from build123d import *

# Parameters (mm, degrees)
F0_R     = 26.071284
F1_DEPTH = 25.4


with BuildPart() as f1:
    # F0 (on Front) → F1 (new body)
    with BuildSketch(Plane.XZ):
        with BuildLine():
            Line((-40.295284, 43.9585), (-40.295284, -43.9585))
            Line((-40.295284, -43.9585), (40.295284, -43.9585))
            Line((40.295284, -43.9585), (40.295284, 43.9585))
            ThreePointArc((40.295284, 43.9585), (0, 3.663216), (-40.295284, 43.9585))
        make_face()
        with BuildLine():
            ThreePointArc((40.295284, 43.9585), (0, 84.253784), (-40.295284, 43.9585))
            ThreePointArc((-40.295284, 43.9585), (0, 3.663216), (40.295284, 43.9585))
        make_face()
        with Locations((0, 43.9585)):
            Circle(F0_R, mode=Mode.SUBTRACT)
    extrude(amount=F1_DEPTH)


solid = f1.part
Geometry: final body of the model. Coordinates: model frame, mm. Round coordinates to 2 decimals unless told otherwise and drop trailing zeros. Loops run counter-clockwise (first coordinate to the right, second up) from the corner with the lowest first, then second, coordinate; pieces in that order, holes last. Notation, with made-up numbers: M 7.25,-13.5 L 52.25,-13.5 A15 ccw 52.25,13.5 Z; hole C 47,-24 d2. An arc over 180 degrees is marked long. One line per question, with ' | ' between items.
(1) Cut plane D-D on x = 29. Return the cut outline in (y, z).
Check result:
outline: M -25.4,-43.96 L 0,-43.96 L 0,71.94 L -25.4,71.94 Z
(2) Cut plane C-C on y = -20.75. Return the cut outline in (x, z), plus the area to 3 significant figures.
Check result:
outline: M -40.3,-43.96 L 40.3,-43.96 L 40.3,43.96 A40.3 ccw -40.3,43.96 Z; hole C 0,43.96 d52.14 | area: 7,500 mm2
(3) Material intervals for line 1 along X through (y, z) = (-1.5, 43); line 2 along Z through (x, y) = (0, -11); line 3 along Z through (x, y) = (12, -14), sorted ascending. Write a range as from..to.
Check result:
line 1: x = -40.3..-26.05, 26.05..40.3 | line 2: z = -43.96..17.89, 70.03..84.25 | line 3: z = -43.96..20.81, 67.1..82.43
(4) Cut plane B-B on z = 21. Return the cut outline in (x, y), plus the area to 3 significant figures.
Check result:
outline: M -40.3,-25.4 L -12.35,-25.4 L -12.35,0 L -40.3,0 Z; M 12.35,-25.4 L 40.3,-25.4 L 40.3,0 L 12.35,0 Z | area: 1,420 mm2
(5) Pull-direction query (Z, two-part tool) for faces 1 (the flat face through (-1, -13, -43.958)), 2 (the flat face through (-1, 0, 7)), 3 (the cylindrical face through (14.02, -12.52, 65.94)); classes: +Z half, -Z half, draft (parallel to the pull), parting line (faces both ways), or undercut.
Check result:
face 1: -Z half | face 2: draft | face 3: undercut
(6) Contact query for flat-ended pins moving along their axis: P1, Ø2, axis at x = 26.5, y = -12, coming from the +Z side; P2, Ø1.5, axis at x = -31.5, y = -11.5, coming from the +Z side; P3, Ø12, axis at x = -31, y = -13.5, coming from the +Z side. Output: stop coordinate, or through.
Check result:
P1: stops at z = 75.16 | P2: stops at z = 70 | P3: stops at z = 75.56
(7) Cut plane A-A on x = 0. Return the cut outline in (y, z).
Check result:
outline: M -25.4,-43.96 L 0,-43.96 L 0,17.89 L -25.4,17.89 Z; M -25.4,70.03 L 0,70.03 L 0,84.25 L -25.4,84.25 Z
